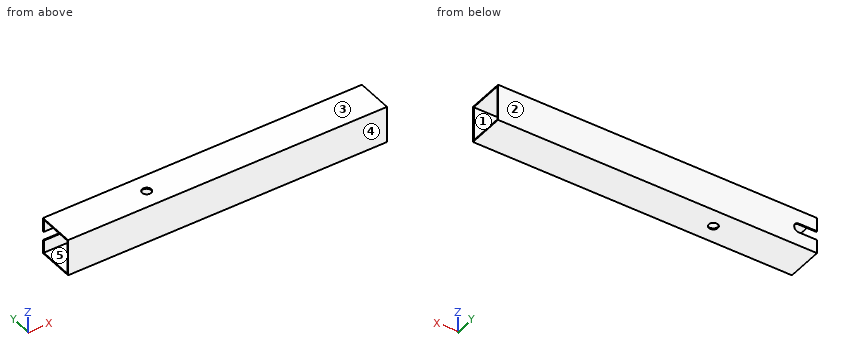
Autodesk Inventor part; units mm, degrees
ref_plane "YZ Plane" through (0, 0, 0) normal (1, 0, 0) x (0, 1, 0)
ref_plane "XZ Plane" through (0, 0, 0) normal (0, 1, 0) x (-1, 0, 0)
ref_plane "XY Plane" through (0, 0, 0) normal (0, 0, 1) x (1, 0, 0)
sketch "Sketch2" plane through (0, 0, 0) normal (0, 0, 1) x (1, 0, 0)
  circle A0 centre (0, 0) radius 12.7
  line L0 (12.7, 0) -> (635, 0)
  line L1 (635, 0) -> (635, 50.8)
  line L2 (635, 50.8) -> (0, 50.8)
  line L3 (0, 50.8) -> (0, 12.7)
  line L4 (635, 0) -> (635, -50.8)
  line L5 (635, -50.8) -> (0, -50.8)
  line L6 (0, -50.8) -> (0, -12.7)
  line L7 (-12.7, 0) -> (-254, 0)
  line L8 (-254, 0) -> (-254, 50.8)
  line L9 (-254, 50.8) -> (0, 50.8)
  line L10 (0, 50.8) -> (0, 12.7)
  line L11 (0, -50.8) -> (0, -12.7)
  line L12 (-254, 0) -> (-254, -50.8)
  line L13 (-254, -50.8) -> (0, -50.8)
  dimension "d0" = 25.4
  dimension "d1" = 50.8
  dimension "d2" = 635
  dimension "d3" = 254
extrude "Extrusion1" add sketch "Sketch2" along normal mid plane 101.6 contours L0 L4 L5 L6 A0 | A0 L3 L2 L1 L0 | A0 L7 L8 L9 L3 | L6 L13 L12 L7 A0
sketch "Sketch3" plane through (0, 0, 0) normal (1, 0, 0) x (0, 1, 0)
  line L0 (50.8, -50.8) -> (50.8, 50.8)
  line L1 (-50.8, -50.8) -> (50.8, -50.8)
  line L2 (50.8, 50.8) -> (-50.8, 50.8)
  line L3 (-50.8, -50.8) -> (-50.8, 50.8)
  line L4 (-50.8, 50.8) -> (-50.8, -50.8)
  line L5 (-50.8, -50.8) -> (50.8, -50.8)
  line L6 (50.8, -50.8) -> (50.8, 50.8)
  line L7 (50.8, 50.8) -> (-50.8, 50.8)
  line L8 (-50.8, 50.8) -> (50.8, -50.8) construction
  line L9 (-50.8, -50.8) -> (50.8, 50.8) construction
  line L10 (-47.625, 47.625) -> (-47.625, -47.625)
  line L11 (-47.625, -47.625) -> (47.625, -47.625)
  line L12 (47.625, -47.625) -> (47.625, 47.625)
  line L13 (47.625, 47.625) -> (-47.625, 47.625)
  line L14 (-47.625, 47.625) -> (47.625, -47.625) construction
  line L15 (-47.625, -47.625) -> (47.625, 47.625) construction
  line L16 (-12.7, 50.8) -> (-12.7, -50.8)
  point P0 (0, 0)
  point P1 (-12.7, 47.625)
  point P2 (-12.7, -47.625)
  dimension "d6" = 3.175
  dimension "d7" = 3.175
extrude "Extrusion3" cut sketch "Sketch3" along normal through all both and the other way through all contours L16 L13 L12 L11 | L11 L10 L13 L16
sketch "Sketch4" plane through (-254, 50.8, 50.8) normal (0, 1, 0) x (1, 0, 0)
  line L0 (0, 50.8) -> (50.8, 50.8) construction
  line L1 (0, 98.425) -> (0, 3.175)
  line L2 (0, 38.1) -> (50.8, 38.1)
  line L3 (50.8, 63.5) -> (0, 63.5)
  arc A0 (50.8, 38.1) -> (50.8, 63.5) centre (50.8, 50.8) ccw
  line L4 (0, 63.5) -> (0, 38.1)
  point P0 (254, 50.8)
  dimension "d12" = 50.8
  dimension "d13" = 25.4
extrude "SlotForCable" cut sketch "Sketch4" against normal up to surface (3.175 mm away)
equation "\"d2\" = longDistanceFromHole"
equation "\"d3\" = shortDistanceFromHole"
equation "\"materialWidth\" = 101.6"
equation "\"shortDistanceFromHole\" = 254"
equation "\"longDistanceFromHole\" = 635"
properties part number "CatapultArm" material "Aluminum 6061"
Read the model definition and answer for the solid it produces. Units are mm, in the model's axes. Face numbers are marked on the shaded views. A direction names the side the tool comes from. Coordinates: 2 decimals unless noted, no trailing zeros. Order: outer loops, then holes, each group sorted by start corner. A loop starts at its lowest first (then second) coordinate and runs counter-clockwise, first axis right, second up. Notation, with made-up numbers: M -33.5,18 L 1.5,18 A24 cw 1.5,28 Z; hole C 65,-26.5 d11. An arc over 180 degrees is marked long. Put each result on its own line as item: value. Start each with the question number.
Item 1: Consider probe 1 along Z at (x, y) = (598.5, -15) (3 decimals); probe 2 along Y at (x, z) = (0, -48.75); probe 3 along X at (y, z) = (0, 48.7). Determine where each line is inside the solid, lowest interval first. Write a range as [from, to].
Item 2: Section B-B, the plane z = 0 is taken. Determine the outline of the cut face in (x, y) (3 decimals).
Item 3: Section A-A, the plane y = 0 is taken. Determine the outline of the cut face in (x, z) (3 decimals), plus the area to 3 significant figures.
Item 4: The mould has two halves that part along Y. Classify the marked faces 1, 2 and 3: +Y half, -Y half, draft (parallel to the pull), parting line (faces both ways), or undercut.
Item 5: Section C-C, the plane x = 0 is taken. Determine the outline of the cut face in (y, z) (3 decimals).
Item 6: Section D-D, the plane x = 218.5 is taken. Determine the outline of the cut face in (y, z) (3 decimals), plus the area to 3 significant figures.
Item 7: For the marked faces 4 and 5, determine the directions among +Z, -Z, +X, -X, +Y, -Y from which every point of the face is accessible in a straight line to the end or side of a thin tool.
Computed:
1. probe 1: z = [-50.8, -47.625], [47.625, 50.8]
1. probe 2: y = [-50.8, -12.7], [12.7, 50.8]
1. probe 3: x = [-254, -12.7], [12.7, 635]
2. outline: M -254,-50.8 L 635,-50.8 L 635,-47.625 L -254,-47.625 Z; M -190.5,47.625 L 635,47.625 L 635,50.8 L -190.5,50.8 Z
3. outline: M -254,-50.8 L -12.7,-50.8 L -12.7,-47.625 L -254,-47.625 Z; M -254,47.625 L -12.7,47.625 L -12.7,50.8 L -254,50.8 Z; M 12.7,-50.8 L 635,-50.8 L 635,-47.625 L 12.7,-47.625 Z; M 12.7,47.625 L 635,47.625 L 635,50.8 L 12.7,50.8 Z
3. area: 5,480 mm2
4. face 1: undercut
4. face 2: +Y half
4. face 3: draft
5. outline: M -50.8,-50.8 L -12.7,-50.8 L -12.7,-47.625 L -47.625,-47.625 L -47.625,47.625 L -12.7,47.625 L -12.7,50.8 L -50.8,50.8 Z; M 12.7,-50.8 L 50.8,-50.8 L 50.8,50.8 L 12.7,50.8 L 12.7,47.625 L 47.625,47.625 L 47.625,-47.625 L 12.7,-47.625 Z
6. outline: M -50.8,-50.8 L 50.8,-50.8 L 50.8,50.8 L -50.8,50.8 Z; hole M -47.625,-47.625 L 47.625,-47.625 L 47.625,47.625 L -47.625,47.625 Z
6. area: 1,250 mm2
7. face 4: +Z, -Z, +X, -X, -Y
7. face 5: +X, -X
